The model under review builds one solid part; all positions refer to its coordinate system, in mm. A direction names the side the tool comes from. Round coordinates to 2 decimals unless told otherwise and drop trailing zeros. Order: outer loops, then holes, each group sorted by start corner. A loop starts at its lowest first (then second) coordinate and runs counter-clockwise, first axis right, second up.
```python
from build123d import *

# Parameters (mm, degrees)
SHEET_EXTRUDE_1_1_BACK  = 400
SHEET_EXTRUDE_1_1_DEPTH = 400
THICKEN_1_T1            = 0.5
THICKEN_1_T2            = 0.5


with BuildPart() as body_1:
    # Sheet Extrude 1: a surface, the sketch's curves swept straight by 400 mm
    with BuildLine(Plane.XY.offset(-SHEET_EXTRUDE_1_1_BACK), mode=Mode.PRIVATE) as sheet_extrude_1_1_path:
        Line((7, 14.5), (7, 0))
        Line((7, 0), (-7, 0))
        Line((-7, 0), (-7, 14.5))
    sheet_extrude_1_1 = Shell.extrude(sheet_extrude_1_1_path.wire(), (0 * SHEET_EXTRUDE_1_1_DEPTH, 0 * SHEET_EXTRUDE_1_1_DEPTH, 1 * SHEET_EXTRUDE_1_1_DEPTH))
    add(Solid.thicken(sheet_extrude_1_1, THICKEN_1_T1))
    add(Solid.thicken(sheet_extrude_1_1, -THICKEN_1_T2))


solid = body_1.part
```
(1) Consider section B-B (z = -233). Write out the cut boundary in (x, y).
Data:
outline: (-7.5, -0.5) - (7.5, -0.5) - (7.5, 14.5) - (6.5, 14.5) - (6.5, 0.5) - (-6.5, 0.5) - (-6.5, 14.5) - (-7.5, 14.5) - close
(2) Insertion check: pin 1 (2 mm diameter, centred on x = -2.5, z = -293.5, fed in from +Y); pin 2 (6 mm diameter, centred on x = -1.5, y = 6.5, fed in from -Z). Each pin has a flat end and moves straight along its axis. Give the tip position at first contact, or say it passes through.
Data:
pin 1: stops at y = 0.5
pin 2: passes through
(3) Draft analysis for pull direction X (two halves, no side actions). For faces 3 (the flat face through (-7.5, 7, -203)), 4 (the flat face through (0, 0, 0)), 5 (the flat face through (0, 0.5, -203)), 6 (the flat face through (6.5, 8, -203)), state which applies: pulls with the +X half, pulls with the -X half, needs draft (parallel to the pull), parting line crosses it, or undercut.
Data:
face 3: pulls with the -X half
face 4: needs draft
face 5: undercut
face 6: undercut
(4) Consider section A-A (y = 11.5). Write out the cut boundary in (x, z), and give its area (3 significant figures).
Data:
outline: (-7.5, -400) - (-6.5, -400) - (-6.5, 0) - (-7.5, 0) - close; (6.5, -400) - (7.5, -400) - (7.5, 0) - (6.5, 0) - close
area: 800 mm2
(5) To check wall thickness, follow probe 1 along X at (y, z) = (3.5, -193); probe 2 along Y at (x, z) = (0.25, -345). State the ranges of each line that lie inside material, in increasing order.
Data:
probe 1: x = -7.5 to -6.5, 6.5 to 7.5
probe 2: y = -0.5 to 0.5
(6) Consider section C-C (x = 0.25). Write out the cut boundary in (y, z), and give its area (3 significant figures).
Data:
outline: (-0.5, -400) - (0.5, -400) - (0.5, 0) - (-0.5, 0) - close
area: 400 mm2
(7) For faces 1 (the flat face through (-6.5, 7, -203)), 2 (the flat face through (0, 0, -400)), list the 3-axis set-ups (+Z, -Z, +X, -X, +Y, -Y) from which the entire face can be reached by the end or side of a thin tool; tool diameter is ignored.
Data:
face 1: +Z, -Z, +Y
face 2: -Z, +X, -X, +Y, -Y
